Read the model definition and answer for the solid it produces. Units are mm, in the model's axes. Give positions to 0.01 mm unless a question says otherwise; leave off trailing zeros. Order: outer loops, then holes, each group sorted by start corner. A loop starts at its lowest first (then second) coordinate and runs counter-clockwise, first axis right, second up. Notation, with made-up numbers: (80.25, 48.25) - (115.25, 48.25) arc R26 ccw to (115.25, 76.25) - close; hole circle Ø10 at (65.5, -17). An arc over 180 degrees is marked (long way). Write item = value, one per line.
```python
from build123d import *

# Parameters (mm, degrees)
F0_W     = 72
F0_H     = 163
F1_DEPTH = 5
F2_W     = 30
F2_H     = 26
F2_R     = 7.5
F3_DEPTH = 25
F4_R     = 10.8639610307
F5_R     = 5.3112698372


with BuildPart() as f1:
    # F0 (on Top) → F1 (new body)
    with BuildSketch(Plane.XY):
        with Locations((-8.3418504, 45.0741375387)):
            Rectangle(F0_W, F0_H)
    extrude(amount=-F1_DEPTH)

    # F2 (on face) → F3 (cut)
    with BuildSketch(Plane.XY):
        with Locations((12.6581496, 96.5741375387)):
            Rectangle(F2_W, F2_H)
        with Locations((-29.3418504, 96.5741375387)):
            Rectangle(F2_W, F2_H)
        with Locations((12.6581496, 68.5741375387)):
            Circle(F2_R)
        with Locations((-29.3418504, 68.5741375387)):
            Circle(F2_R)
        with Locations((-8.3418504, 38.5741375387)):
            Circle(F2_R)
        with Locations((-29.3418504, -21.4258624613)):
            Circle(F2_R)
        with Locations((12.6581496, -21.4258624613)):
            Circle(F2_R)
    extrude(amount=-F3_DEPTH, mode=Mode.SUBTRACT)

    # F4
    f4_edges = [f1.edges().sort_by_distance(p)[0] for p in [
        (-2.34185, 109.574138, -2.5),
        (-2.34185, 83.574138, -2.5),
        (-14.34185, 83.574138, -2.5),
        (-14.34185, 109.574138, -2.5),
    ]]
    fillet(f4_edges, radius=F4_R)

    # F5
    f5_edges = [f1.edges().sort_by_distance(p)[0] for p in [
        (27.65815, 126.574138, -2.5),
        (-44.34185, 126.574138, -2.5),
        (-44.34185, 109.574138, -2.5),
        (-44.34185, 83.574138, -2.5),
        (27.65815, 109.574138, -2.5),
        (27.65815, 83.574138, -2.5),
        (-44.34185, -36.425862, -2.5),
        (27.65815, -36.425862, -2.5),
    ]]
    fillet(f5_edges, radius=F5_R)


solid = f1.part
```
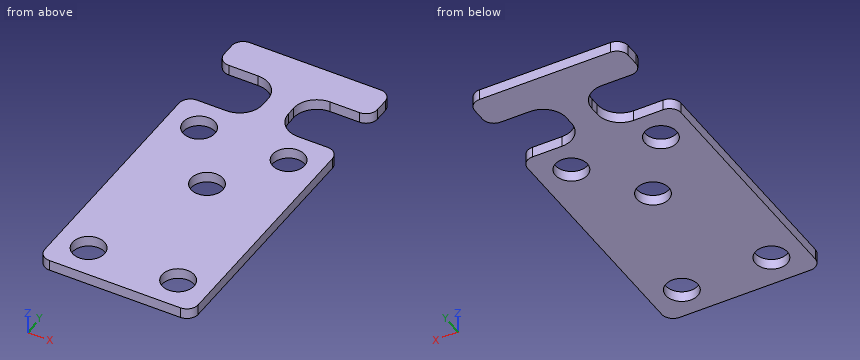
1. Straight lines are drawn through the part: L1, parallel to Y at x = -30, z = -1.95; L2, parallel to Y at x = 14, z = -3.35; L3, parallel to X at y = -18.5, z = -3.7. For each, find the intervals that lie inside material, in ascending order. Write a range as [from, to].
Recorded:
L1 = [-36.43, -28.9], [-13.95, 61.1], [76.05, 83.57], [109.57, 126.57]
L2 = [-36.43, -28.8], [-14.05, 61.2], [75.95, 83.57], [109.57, 126.57]
L3 = [-44.34, -36.25], [-22.44, 5.75], [19.56, 27.66]
2. Section D-D (x = -23.5) is taken. Determine the outline of the cut face in (y, z).
Recorded:
outline = (-36.43, -5) - (-26.13, -5) - (-26.13, 0) - (-36.43, 0) - close; (-16.72, -5) - (63.87, -5) - (63.87, 0) - (-16.72, 0) - close; (73.28, -5) - (83.71, -5) - (83.71, 0) - (73.28, 0) - close; (109.44, -5) - (126.57, -5) - (126.57, 0) - (109.44, 0) - close
3. Section B-B (x = 18.5) is taken. Determine the outline of the cut face in (y, z).
Recorded:
outline = (-36.43, -5) - (-26.13, -5) - (-26.13, 0) - (-36.43, 0) - close; (-16.72, -5) - (63.87, -5) - (63.87, 0) - (-16.72, 0) - close; (73.28, -5) - (83.57, -5) - (83.57, 0) - (73.28, 0) - close; (109.57, -5) - (126.57, -5) - (126.57, 0) - (109.57, 0) - close
4. Section A-A (x = -10) is taken. Determine the outline of the cut face in (y, z), and give its area (3 significant figures).
Recorded:
outline = (-36.43, -5) - (31.26, -5) - (31.26, 0) - (-36.43, 0) - close; (45.89, -5) - (126.57, -5) - (126.57, 0) - (45.89, 0) - close
area = 742 mm^2
5. A flat-ended cylindrical pin translates along its axis: pin 1 (1 mm diameter, centred on y = 104, z = -0.5, fed in from -X). Find the tip coordinate at first contact, or state that the pin passes through.
Recorded:
pin_1 = -16.01
6. Section C-C (z = -1.65) is taken. Count the separate pieces of the cut face and the enclosed holes in it, and give its area (3 significant figures).
Recorded:
separate_pieces = 1
enclosed_holes = 5
area = 9,350 mm^2
